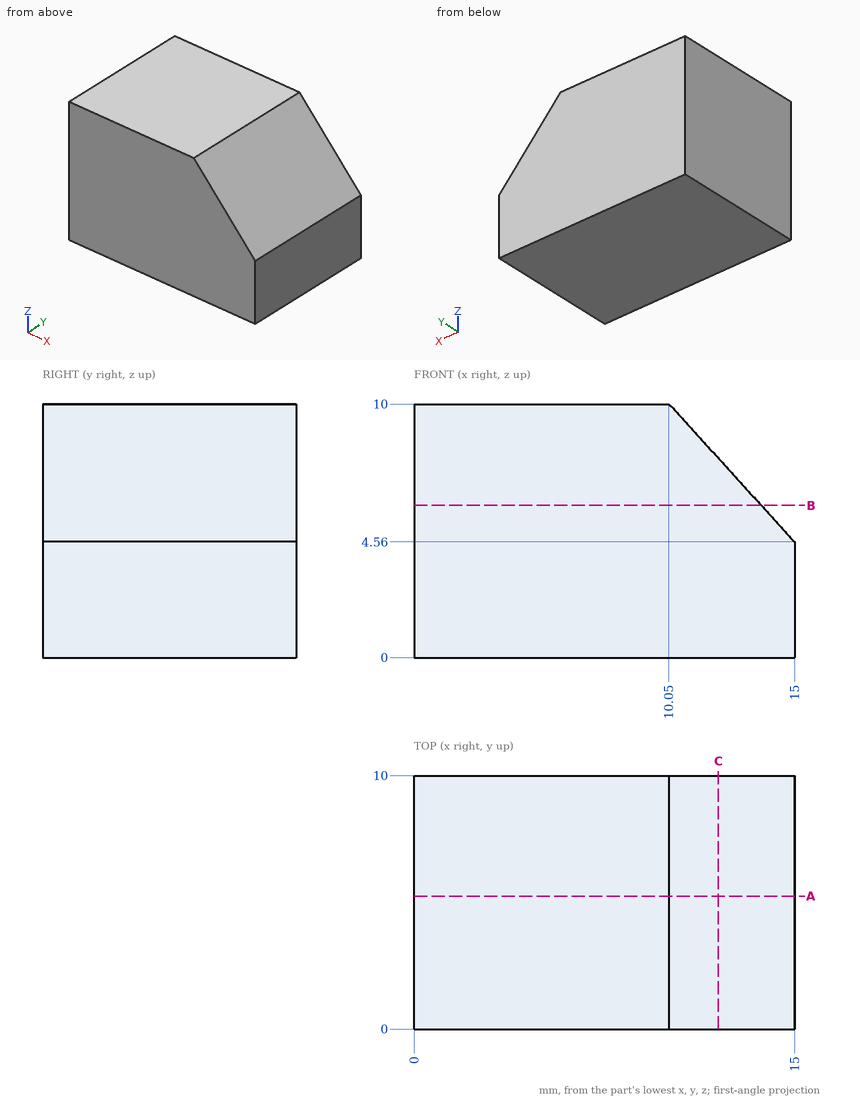
The drawing under review shows one solid part. Ordinate dimensions are in mm from its lowest x, y, z. Coordinates: 2 decimals unless noted, no trailing zeros. Loops run counter-clockwise (first coordinate to the right, second up) from the corner with the lowest first, then second, coordinate; pieces in that order, holes last.
Item 1: Clearance check with a flat-ended pin moving along its axis: pin 1 (1 mm diameter, centred on x = 9, y = 7.5, fed in from -Z). State where the tip first meets the part, or that it passes through.
Completed:
pin 1: stops at z = 0
Item 2: Add section B-B (z = 6). Write out the cut boundary in (x, y).
Completed:
outline: (0, 0) - (13.69, 0) - (13.69, 10) - (0, 10) - close
Item 3: Wall thickness on L1, parallel to Z at x = 14, y = 2; L2, parallel to X at y = 4.5, z = 6.75 (1 decimal); L3, parallel to X at y = 2.5, z = 6: over which ranges is each line inside the solid? List them lowest first.
Completed:
L1: z = 0 to 5.66
L2: x = 0 to 13
L3: x = 0 to 13.69
Item 4: Add section A-A (y = 5.25). Write out the cut boundary in (x, z).
Completed:
outline: (0, 0) - (15, 0) - (15, 4.56) - (10.05, 10) - (0, 10) - close
Item 5: Add section C-C (x = 12). Write out the cut boundary in (y, z).
Completed:
outline: (0, 0) - (10, 0) - (10, 7.86) - (0, 7.86) - close
